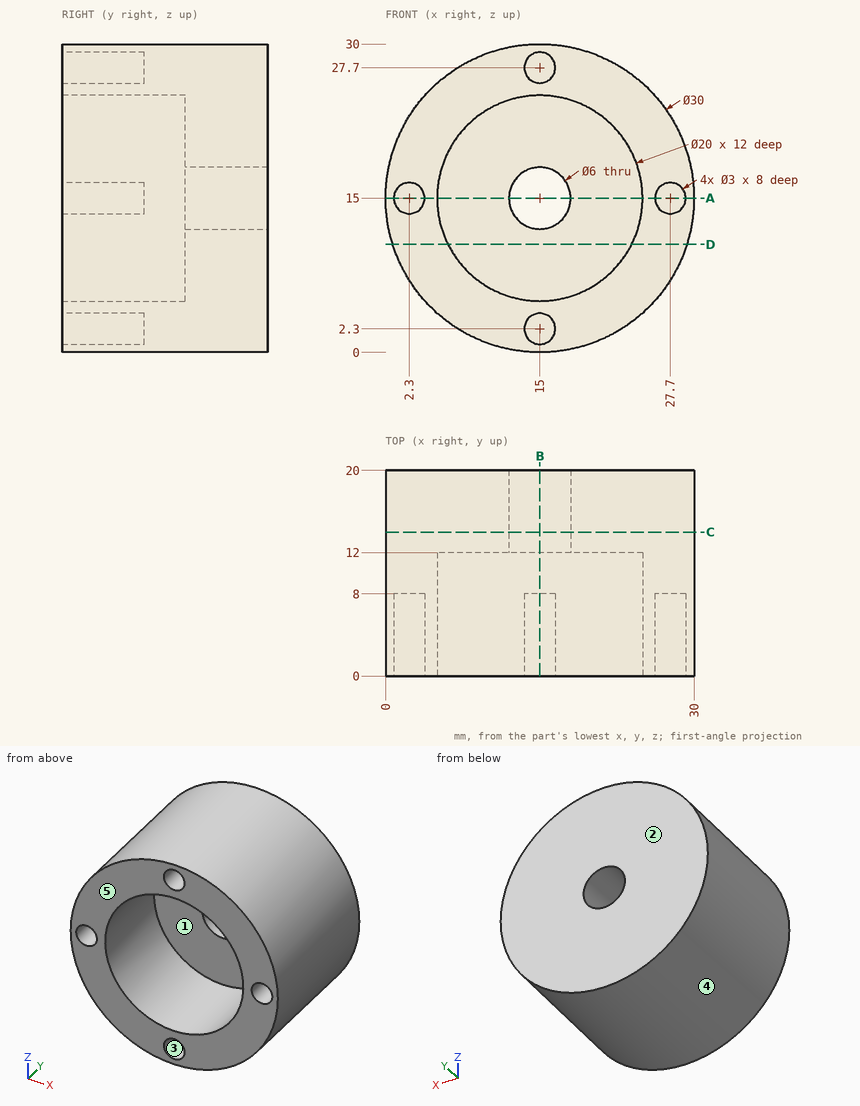
Check sheet for the drawn part. Datum: minimum x, y, z corner. Units: mm. A direction names the side the tool comes from. Give positions to 0.01 mm unless a question says otherwise; leave off trailing zeros. Order: outer loops, then holes, each group sorted by start corner. A loop starts at its lowest first (then second) coordinate and runs counter-clockwise, first axis right, second up. Notation, with made-up numbers: (-28.75, -30) - (7.25, -30) arc R29 ccw to (7.25, -1) - close; hole circle Ø9 at (7, 58). An arc over 180 degrees is marked (long way). Write item = value, one per line. Start each with the question number.
1) Section check D-D (z = 10.5). Enter the section's corners in (x, y).
2) Draft check along Z on the marked faces 3, 4 and 5. Enter one of: released by +Z, released by -Z, zero draft, split by the parting line, or undercut.
3) Section check A-A (z = 15). Enter the section's corners in (x, y), then the cut area to 3 significant figures.
4) Section check C-C (y = 14). Enter the section's corners in (x, z), then the cut area to 3 significant figures.
5) Scan lines: L1, parallel to X at y = 2, z = 15; L2, parallel to Z at x = 14, y = 4.25; L3, parallel to Y at x = 8.5, z = 20.5. Record each from-to range of solid material in increasing order.
6) Gauge pin test, flat ends, axial feed: pin 1 Ø0.9 at (x, z) = (2.5, 15.5) entering from -Y; pin 2 Ø1.5 at (x, y) = (25.5, 6.5) entering from +Z; pin 3 Ø12 at (y, z) = (8.5, 3.5) entering from +X; pin 4 Ø5.5 at (x, z) = (15, 15) entering from -Y. Record the tip position at first contact, or that the pin passes through.
7) Section check B-B (x = 15). Enter the section's corners in (y, z).
8) Access from +Z, -Z, +X, -X, +Y, -Y to the whole of each face (thin tool, end or side, straight path). Record for the marked faces 1 and 2.
Geometry check:
q1.outline = (0.69, 0) - (6.07, 0) - (6.07, 12) - (23.93, 12) - (23.93, 0) - (29.31, 0) - (29.31, 20) - (0.69, 20) - close
q2.face_3 = undercut
q2.face_4 = split by the parting line
q2.face_5 = zero draft
q3.outline = (0, 0) - (0.8, 0) - (0.8, 8) - (3.8, 8) - (3.8, 0) - (5, 0) - (5, 12) - (12, 12) - (12, 20) - (0, 20) - close; (18, 12) - (25, 12) - (25, 0) - (26.2, 0) - (26.2, 8) - (29.2, 8) - (29.2, 0) - (30, 0) - (30, 20) - (18, 20) - close
q3.area = 264 mm2
q4.outline = circle Ø30 at (15, 15); hole circle Ø6 at (15, 15)
q4.area = 679 mm2
q5.L1 = 0 to 0.8, 3.8 to 5, 25 to 26.2, 29.2 to 30
q5.L2 = 0.03 to 1.18, 3.42 to 5.05, 24.95 to 26.58, 28.82 to 29.97
q5.L3 = 12 to 20
q6.pin_1 = 8
q6.pin_2 = 26.4
q6.pin_3 = 28.96
q6.pin_4 = through
q7.outline = (0, 0) - (20, 0) - (20, 12) - (12, 12) - (12, 5) - (0, 5) - (0, 3.8) - (8, 3.8) - (8, 0.8) - (0, 0.8) - close; (0, 25) - (12, 25) - (12, 18) - (20, 18) - (20, 30) - (0, 30) - (0, 29.2) - (8, 29.2) - (8, 26.2) - (0, 26.2) - close
q8.face_1 = -Y
q8.face_2 = +Z, -Z, +X, -X, +Y
